The model under review builds one solid part; all positions refer to its coordinate system, in mm. A direction names the side the tool comes from. Round coordinates to 2 decimals unless told otherwise and drop trailing zeros. Loops run counter-clockwise (first coordinate to the right, second up) from the corner with the lowest first, then second, coordinate; pieces in that order, holes last. Notation, with made-up numbers: (13, 16.25) -> (59, 16.25) arc R24 ccw to (59, 46.25) -> close; hole circle Ø5 at (-22.5, -28.5). An arc over 180 degrees is marked (long way). Return JSON: item names as keys, results as strings. Group by question number.
```python
from build123d import *

# Parameters (mm, degrees)
EXTRUDE_1_DEPTH     = 5
EXTRUDE_2_DEPTH     = 10
SKETCH_3_R          = 3
CUT_EXTRUDE_1_DEPTH = 2.6
SKETCH_4_R          = 2
CUT_EXTRUDE_2_DEPTH = 37.149135536
SKETCH_5_R          = 6
CUT_EXTRUDE_3_DEPTH = 10
SKETCH_6_R          = 1.5
CUT_EXTRUDE_4_DEPTH = 36.397740041


with BuildPart() as part:
    # 草图1 → 凸台-拉伸1 (new body)
    with BuildSketch(Plane.XY):
        with BuildLine():
            Line((0, 8), (25, 8))
            ThreePointArc((25, 8), (33, 0), (25, -8))
            Line((25, -8), (0, -8))
            ThreePointArc((0, -8), (-8, 0), (0, 8))
        make_face()
    extrude(amount=EXTRUDE_1_DEPTH)

    # 草图2 → 凸台-拉伸2 (add)
    with BuildSketch(Plane.XY.offset(5)):
        with BuildLine():
            Line((4.950165565, -8), (20.049834435, -8))
            ThreePointArc((20.049834435, -8), (23.5, 0), (20.049834435, 8))
            Line((20.049834435, 8), (4.950165565, 8))
            ThreePointArc((4.950165565, 8), (1.5, 0), (4.950165565, -8))
        make_face()
    extrude(amount=EXTRUDE_2_DEPTH)

    # 草图3 → 切除-拉伸1 (cut)
    with BuildSketch(Plane.XY.offset(15)):
        with Locations((12.5, 0)):
            Circle(SKETCH_3_R)
    extrude(amount=-CUT_EXTRUDE_1_DEPTH, mode=Mode.SUBTRACT)

    # 草图4 → 切除-拉伸2 (cut, through all)
    with BuildSketch(Plane.XY.offset(12.4)):
        with Locations((12.5, 0)):
            Circle(SKETCH_4_R)
    extrude(amount=-CUT_EXTRUDE_2_DEPTH, mode=Mode.SUBTRACT)

    # 草图5 → 切除-拉伸3 (cut)
    with BuildSketch(Plane(origin=(0, 0, 0), x_dir=(-1, 0, 0), z_dir=(0, 0, -1))):
        with Locations((-12.5, 0)):
            Circle(SKETCH_5_R)
    extrude(amount=-CUT_EXTRUDE_3_DEPTH, mode=Mode.SUBTRACT)

    # 草图6 → 切除-拉伸4 (cut, through all)
    with BuildSketch(Plane.XY.offset(5)):
        with Locations((-2.5, 0)):
            Circle(SKETCH_6_R)
        with Locations((27.5, 0)):
            Circle(SKETCH_6_R)
    extrude(amount=-CUT_EXTRUDE_4_DEPTH, mode=Mode.SUBTRACT)


solid = part.part
```
1. We need section C-C, the plane y = 0.5. Write out the cut boundary in (x, z), then the cut area to 3 significant figures.
2. We need section D-D, the plane z = 8.5. Write out the cut boundary in (x, y).
3. Tool access review of faces 5 (the face through (10, 0, 12.4)), 6 (the face through (1.5, 0.1, 9.9)), 7 (the face through (6.777, 1.802, 4.93)): name each direction out of +Z, -Z, +X, -X, +Y, -Y from which nothing blocks a thin tool from reaching the whole face with its end or side.
4. Draft analysis for pull direction Y (two halves, no side actions). For faces 1 (the face through (10.9, -1.2, 11.2)), 2 (the face through (12, 8, 6)), 3 (the face through (26, 0, 3)), 4 (the face through (10, -2, 15)), state which applies: pulls with the +Y half, pulls with the -Y half, needs draft (parallel to the pull), parting line crosses it, or undercut.
5. For P1, Ø2, axis at x = -3.5, z = 7.5, coming from the -Y side; P2, Ø3, axis at x = 1, z = 9, coming from the -Y side; P3, Ø1.5, axis at x = 10, y = -2.5, coming from the -Z side; P4, Ø8, axis at y = 3.5, z = 11, coming from the -X side, all flat-tipped, find the tip position at first contact; note any pin that passes through.
6. We need section A-A, the plane x = 12.5. Write out the cut boundary in (y, z), then the cut area to 3 significant figures.
7. Wall thickness on line 1 (Y direction, x = 12.5, z = 4.5); line 2 (Y direction, x = 12.5, z = 10.5); line 3 (Z direction, x = 30, y = -2.25): over which ranges is each line inside the solid? List them lowest first.
8. We need section B-B, the plane z = 2. Write out the cut boundary in (x, y), then the cut area to 3 significant figures.
Check sheet entries:
{
 "1": {"outline": "(-7.98, 0) -> (-3.91, 0) -> (-3.91, 5) -> (-7.98, 5) -> close; (-1.09, 0) -> (6.52, 0) -> (6.52, 10) -> (10.56, 10) -> (10.56, 12.4) -> (9.54, 12.4) -> (9.54, 15) -> (1.51, 15) -> (1.51, 5) -> (-1.09, 5) -> close; (14.44, 10) -> (18.48, 10) -> (18.48, 0) -> (26.09, 0) -> (26.09, 5) -> (23.49, 5) -> (23.49, 15) -> (15.46, 15) -> (15.46, 12.4) -> (14.44, 12.4) -> close; (28.91, 0) -> (32.98, 0) -> (32.98, 5) -> (28.91, 5) -> close", "area": "252 mm²"},
 "2": {"outline": "(4.95, -8) -> (20.05, -8) arc R11 ccw to (20.05, 8) -> (4.95, 8) arc R11 ccw to start; hole circle Ø12 at (12.5, 0)"},
 "3": {"face 5": "+Z", "face 6": "+Z, -X", "face 7": "-Z"},
 "4": {"face 1": "undercut", "face 2": "pulls with the +Y half", "face 3": "undercut", "face 4": "needs draft"},
 "5": {"P1": "passes through", "P2": "stops at y = -4.58", "P3": "stops at z = 10", "P4": "stops at x = 1.5"},
 "6": {"outline": "(-8, 0) -> (-6, 0) -> (-6, 10) -> (-2, 10) -> (-2, 12.4) -> (-3, 12.4) -> (-3, 15) -> (-8, 15) -> close; (2, 10) -> (6, 10) -> (6, 0) -> (8, 0) -> (8, 15) -> (3, 15) -> (3, 12.4) -> (2, 12.4) -> close", "area": "94.8 mm²"},
 "7": {"line 1": "y = -8 to -6, 6 to 8", "line 2": "y = -8 to -2, 2 to 8", "line 3": "z = 0 to 5"},
 "8": {"outline": "(0, -8) -> (25, -8) arc R8 ccw to (25, 8) -> (0, 8) arc R8 ccw to start; hole circle Ø3 at (-2.5, 0); hole circle Ø12 at (12.5, 0); hole circle Ø3 at (27.5, 0)", "area": "474 mm²"}
}
